Autodesk Fusion 360 part; units mm, degrees
sketch "Sketch1" plane through (0, 0, 0) normal (0, 0, 1) x (1, 0, 0)
  line L0 (0, 0) -> (30, 0)
  line L1 (30, 0) -> (30, -30)
  line L2 (30, -30) -> (0, -30)
  line L3 (0, -30) -> (0, 0)
  dimension "d5" = 30
  dimension "d6" = 30
extrude "Extrude1" add sketch "Sketch1" along normal blind 5
sketch "Sketch2" plane through (0, 0, 5) normal (0, 0, 1) x (-1, 0, 0)
  line L0 (0, 30) -> (-30, 30)
  line L1 (-30, 30) -> (-30, 0)
  line L2 (-30, 0) -> (0, 0)
  line L3 (0, 0) -> (0, 30)
  line L4 (0, 0) -> (-30, 0)
  line L5 (-30, 0) -> (-30, 10)
  line L6 (-30, 10) -> (0, 10)
  line L7 (0, 10) -> (0, 0)
  dimension "d10" = 10
  dimension "d11" = 30
extrude "Extrude2" add sketch "Sketch2" along normal blind 35 contours L1 L2 L3 L4 L5 L6 L7
equation "base_sides = 30 mm"
equation "height = 40 mm"
equation "upper_length = 30 mm"
equation "upper_width = 10 mm"
equation "d5 = base_sides"
equation "d6 = base_sides"
equation "base_height = 5 mm"
equation "d8 = base_height"
equation "d10 = upper_width"
equation "d11 = upper_length"
equation "d12 = height - base_height"
Geometry: final body of the model. Coordinates: model frame, mm. A direction names the side the tool comes from. Round coordinates to 2 decimals unless told otherwise and drop trailing zeros. Loops run counter-clockwise (first coordinate to the right, second up) from the corner with the lowest first, then second, coordinate; pieces in that order, holes last.
Item 1: Contact query for flat-ended pins moving along their axis: P1, Ø15, axis at x = 8.5, z = 20, coming from the -Y side; P2, Ø12, axis at x = 19, y = -6, coming from the -Z side; P3, Ø4, axis at x = 16, y = -14, coming from the +Z side. Output: stop coordinate, or through.
Checked values:
P1: stops at y = -10
P2: stops at z = 0
P3: stops at z = 5
Item 2: Section A-A, the plane x = 9.5. Output: boundary loops of the cut face in (y, z), plus the area to 3 significant figures.
Checked values:
outline: (-30, 0) - (0, 0) - (0, 40) - (-10, 40) - (-10, 5) - (-30, 5) - close
area: 500 mm2
Item 3: Section C-C, the plane z = 37. Output: boundary loops of the cut face in (x, y), plus the area to 3 significant figures.
Checked values:
outline: (0, -10) - (30, -10) - (30, 0) - (0, 0) - close
area: 300 mm2
Item 4: Line query: L1, parallel to Z at x = 5.25, y = -26; L2, parallel to Y at x = 11.5, z = 24. Output: solid intervals per line, ascending.
Checked values:
L1: z = 0 to 5
L2: y = -10 to 0
Item 5: Reachability of faces 1 (the flat face through (15, -30, 2)), 2 (the flat face through (15, -10, 22)) from +Z, -Z, +X, -X, +Y, -Y: full face, straight path, thin tool, end or side. Return the list, or none.
Checked values:
face 1: +Z, -Z, +X, -X, -Y
face 2: +Z, +X, -X, -Y
Item 6: Section B-B, the plane y = -12.5. Output: boundary loops of the cut face in (x, z), plus the area to 3 significant figures.
Checked values:
outline: (0, 0) - (30, 0) - (30, 5) - (0, 5) - close
area: 150 mm2
